Model file for the job. Use its own axes, mm. Coordinates: 2 decimals unless noted, no trailing zeros. Order: outer loops, then holes, each group sorted by start corner. A loop starts at its lowest first (then second) coordinate and runs counter-clockwise, first axis right, second up.
from build123d import *

# Parameters (mm, degrees)
SKETCH1_W           = 50.8
SKETCH1_H           = 76.2
SKETCH1_R           = 15.24
SKETCH1_R_2         = 7.62
BOSS_EXTRUDE1_DEPTH = 101.6
FILLET1_R           = 6.35


with BuildPart() as part:
    # Sketch1 → Boss-Extrude1 (new body)
    with BuildSketch(Plane.YZ):
        Rectangle(SKETCH1_W, SKETCH1_H)
        with Locations(Location((0, -7.62, 0), (0, 0, 270))):
            Circle(SKETCH1_R, mode=Mode.SUBTRACT)
        with Locations(Location((0, 22.86, 0), (0, 0, 270))):
            Circle(SKETCH1_R_2, mode=Mode.SUBTRACT)
    extrude(amount=BOSS_EXTRUDE1_DEPTH)

    # Fillet1
    fillet1_edges = [part.edges().sort_by_distance(p)[0] for p in [
        (50.8, -25.4, 38.1),
        (50.8, -25.4, -38.1),
    ]]
    fillet(fillet1_edges, radius=FILLET1_R)


solid = part.part
Q1. Cut at D-D, the plane y = -14. List the corners of the cut face in (x, z), plus the area to 3 significant figures.
Established:
outline: (0, -38.1) - (101.6, -38.1) - (101.6, -13.64) - (0, -13.64) - close; (0, -1.6) - (101.6, -1.6) - (101.6, 38.1) - (0, 38.1) - close
area: 6,520 mm2
Q2. Mould opens along Z. For faces 1 (the face through (50.089, 0.335, 30.473)), 2 (the face through (51.51, -23.59, -36.19)), 3 (the face through (50, 25.4, -1)) say: pulls with the +Z half, pulls with the -Z half, needs draft (parallel to the pull), parting line crosses it, or undercut.
Established:
face 1: undercut
face 2: pulls with the -Z half
face 3: needs draft
Q3. Cut at A-A, the plane z = -7.62. List the corners of the cut face in (x, y), plus the area to 3 significant figures.
Established:
outline: (0, -25.4) - (101.6, -25.4) - (101.6, -15.24) - (0, -15.24) - close; (0, 15.24) - (101.6, 15.24) - (101.6, 25.4) - (0, 25.4) - close
area: 2,060 mm2
Q4. Probe line 1 (Y direction, x = 21.5, z = -7.62); line 2 (Z direction, x = 42.5, y = -4); line 3 (Z direction, x = 9.5, y = 4.5). List the from-to ranges inside material, lowest first.
Established:
line 1: y = -25.4 to -15.24, 15.24 to 25.4
line 2: z = -38.1 to -22.33, 7.09 to 16.37, 29.35 to 38.1
line 3: z = -38.1 to -22.18, 6.94 to 16.71, 29.01 to 38.1
Q5. Cut at B-B, the plane y = 0. List the corners of the cut face in (x, z), plus the area to 3 significant figures.
Established:
outline: (0, -38.1) - (101.6, -38.1) - (101.6, -22.86) - (0, -22.86) - close; (0, 7.62) - (101.6, 7.62) - (101.6, 15.24) - (0, 15.24) - close; (0, 30.48) - (101.6, 30.48) - (101.6, 38.1) - (0, 38.1) - close
area: 3,100 mm2
Q6. Cut at C-C, the plane x = 54. List the corners of the cut face in (y, z).
Established:
outline: (-25.4, -31.75) arc R6.35 ccw to (-19.05, -38.1) - (25.4, -38.1) - (25.4, 38.1) - (-19.05, 38.1) arc R6.35 ccw to (-25.4, 31.75) - close; hole circle Ø30.48 at (0, -7.62); hole circle Ø15.24 at (0, 22.86)
